Check sheet for the modelled part. Datum: model origin and axes. Units: mm. A direction names the side the tool comes from. Coordinates: 2 decimals unless noted, no trailing zeros. Write each loop counter-clockwise with the first axis right and the second up, starting at its lowest first coordinate (ties: lowest second). Pieces come first, ordered by that corner, then holes. Notation, with made-up numbers: M -34,64 L 4,64 A11 cw 4,74 Z; hole C 81,-21 d6. An arc over 180 degrees is marked long. Answer as CSV lines item,"result". Start each with the question number.
Q1. Sectioned sample at C-C, the plane z = 1.7. Record the cut outline in (x, y).
Q2. Sectioned sample at B-B, the plane x = -11. Record the cut outline in (y, z), then the cut area to 3 significant figures.
Q3. Thickness scan on line 1 along X through (y, z) = (-4.75, 0.85); line 2 along Y through (x, z) = (-15, 1.9); line 3 along X through (y, z) = (12.5, 3). Record the ranges inside material, lowest first. Write a range as from..to.
Q4. Sectioned sample at A-A, the plane y = 6.25. Record the cut outline in (x, z), then the cut area to 3 significant figures.
Q5. Access from +Z, -Z, +X, -X, +Y, -Y to the whole of each face (thin tool, end or side, straight path). Record for faces 1 (the flat face through (-21, 11, 1)), 2 (the flat face through (-21.25, -1, 1)), 3 (the flat face through (21.25, -1, 1)).
Q6. Depth check by flat-ended pin: pin 1 Ø0.8 at (x, z) = (6.5, 1) entering from +Y; pin 2 Ø2 at (y, z) = (2, 1) entering from -X; pin 3 Ø1.2 at (y, z) = (5, 1) entering from +X. Enter the tip coordinate at first touch or a pass-through.
from build123d import *

# Parameters (mm, degrees)
F0_W     = 42.5
F0_H     = 23.5
F1_DEPTH = 2.5
F2_W     = 42.5
F2_H     = 23.5
F3_DEPTH = 2
F4_SIZE  = 1
F5_R     = 2


with BuildPart() as f1:
    # F0 (on Top) → F1 (new body)
    with BuildSketch(Plane.XY):
        Rectangle(F0_W, F0_H)
    extrude(amount=F1_DEPTH)

    # F2 (on face) + F0 (on Top) → F3 (join)
    with BuildSketch(Plane.XY.offset(2.5)):
        Polygon((-23.75, 14.25), (-23.75, -11.75), (-21.25, -11.75), (-21.25, 11.75), (21.25, 11.75), (21.25, -11.75), (23.75, -11.75), (23.75, 14.25), align=None)
        Rectangle(F2_W, F2_H)
    with BuildSketch(Plane.XY):
        Rectangle(F0_W, F0_H)
    extrude(amount=F3_DEPTH)

    # F4
    f4_edges = [f1.edges().sort_by_distance(p)[0] for p in [
        (21.25, 11.75, 1.25),
        (-21.25, 11.75, 1.25),
    ]]
    chamfer(f4_edges, length=F4_SIZE)

    # F5
    f5_edges = [f1.edges().sort_by_distance(p)[0] for p in [
        (23.75, 14.25, 3.5),
        (23.75, -11.75, 3.5),
        (-23.75, 14.25, 3.5),
        (-23.75, -11.75, 3.5),
    ]]
    fillet(f5_edges, radius=F5_R)


solid = f1.part
Output:
1,outline,"M -21.25,-11.75 L 21.25,-11.75 L 21.25,10.75 L 20.25,11.75 L -20.25,11.75 L -21.25,10.75 Z"
2,outline,"M -11.75,0 L 11.75,0 L 11.75,2.5 L 14.25,2.5 L 14.25,4.5 L -11.75,4.5 Z"
2,area,"111 mm^2"
3,line 1,"x = -21.25..21.25"
3,line 2,"y = -11.75..11.75"
3,line 3,"x = -23.73..23.73"
4,outline,"M -23.75,2.5 L -21.25,2.5 L -21.25,0 L 21.25,0 L 21.25,2.5 L 23.75,2.5 L 23.75,4.5 L -23.75,4.5 Z"
4,area,"201 mm^2"
5,face 1,"-Z, -X, +Y"
5,face 2,"-Z, -X, +Y, -Y"
5,face 3,"-Z, +X, +Y, -Y"
6,pin 1,"stops at y = 11.75"
6,pin 2,"stops at x = -21.25"
6,pin 3,"stops at x = 21.25"
